Source: CAD feature listing. Evaluate the final solid. Frame: model axes, mm. A direction names the side the tool comes from. Round coordinates to 2 decimals unless told otherwise and drop trailing zeros. Write each loop counter-clockwise with the first axis right and the second up, starting at its lowest first coordinate (ties: lowest second). Pieces come first, ordered by that corner, then holes.
```python
from build123d import *

# Parameters (mm, degrees)
SKETCH1_R           = 2.15
BOSS_EXTRUDE1_DEPTH = 1.5
SKETCH3_W           = 5
SKETCH3_H           = 20
BOSS_EXTRUDE3_DEPTH = 12.5
BOSS_EXTRUDE4_REACH = 52.014


with BuildPart() as part:
    # Sketch1 → Boss-Extrude1 (new, symmetric)
    with BuildSketch(Plane(origin=(0, 0, 0), x_dir=(1, 0, 0), z_dir=(0, 1, 0))):
        with BuildLine():
            Line((-7, -6.25), (7, -6.25))
            ThreePointArc((7, -6.25), (10.535533906, -4.785533906), (12, -1.25))
            Line((12, -1.25), (12, 1.25))
            ThreePointArc((12, 1.25), (10.535533906, 4.785533906), (7, 6.25))
            Line((7, 6.25), (-7, 6.25))
            ThreePointArc((-7, 6.25), (-10.535533906, 4.785533906), (-12, 1.25))
            Line((-12, 1.25), (-12, -1.25))
            ThreePointArc((-12, -1.25), (-10.535533906, -4.785533906), (-7, -6.25))
        make_face()
        with Locations(Location((-7.25, 0, 0), (0, 0, 270))):
            Circle(SKETCH1_R, mode=Mode.SUBTRACT)
        with Locations(Location((7.25, 0, 0), (0, 0, 270))):
            Circle(SKETCH1_R, mode=Mode.SUBTRACT)
    extrude(amount=BOSS_EXTRUDE1_DEPTH, both=True)

    # Sketch3 → Boss-Extrude3 (add)
    with BuildSketch(Plane.XY.offset(6.25)):
        with Locations((0, 11.5)):
            Rectangle(SKETCH3_W, SKETCH3_H)
    extrude(amount=-BOSS_EXTRUDE3_DEPTH)

    # Sketch4 → Revolve1 (revolve)
    with BuildSketch(Plane.XY, mode=Mode.PRIVATE) as revolve1_sk:
        Polygon((-2.5, 19.5), (-22.5, 39.5), (-22.5, 60.085786438), (-21.085786438, 60.085786438), (-21.085786438, 40.085786438), (-2.5, 21.5), (0, 21.5), (0, 19.5), align=None)
    revolve(revolve1_sk.sketch.rotate(Axis((0, 0, 0), (0, 1, 0)), 56.251031305), axis=Axis((0, 0, 0), (0, 1, 0)))

    # Sketch5 → Boss-Extrude4 (add, up to next)
    with BuildSketch(Plane(origin=(0, 21.5, 0), x_dir=(1, 0, 0), z_dir=(0, 1, 0)), mode=Mode.PRIVATE) as boss_extrude4_sk1:
        with BuildLine():
            Line((2.5, -6.25), (2.5, -3.741657387))
            ThreePointArc((2.5, -3.741657387), (0, -4.5), (-2.5, -3.741657387))
            Line((-2.5, -3.741657387), (-2.5, -6.25))
            Line((-2.5, -6.25), (2.5, -6.25))
        make_face()
    boss_extrude4_tool1 = extrude(boss_extrude4_sk1.sketch, amount=BOSS_EXTRUDE4_REACH, mode=Mode.PRIVATE) - part.part
    # Sketch5 → Boss-Extrude4 (add, up to next)
    with BuildSketch(Plane(origin=(0, 21.5, 0), x_dir=(1, 0, 0), z_dir=(0, 1, 0)), mode=Mode.PRIVATE) as boss_extrude4_sk2:
        with BuildLine():
            Line((-2.5, 6.25), (-2.5, 3.741657387))
            ThreePointArc((-2.5, 3.741657387), (0, 4.5), (2.5, 3.741657387))
            Line((2.5, 3.741657387), (2.5, 6.25))
            Line((2.5, 6.25), (-2.5, 6.25))
        make_face()
    boss_extrude4_tool2 = extrude(boss_extrude4_sk2.sketch, amount=BOSS_EXTRUDE4_REACH, mode=Mode.PRIVATE) - part.part
    add(boss_extrude4_tool1.solids().sort_by_distance((0, 21.5, 5.24074))[0])
    add(boss_extrude4_tool2.solids().sort_by_distance((0, 21.5, -5.24074))[0])


solid = part.part
```
Q1. Line query: line 1 (X direction, y = 0, z = 0); line 2 (X direction, y = 53.5, z = 0). Output: solid intervals per line, ascending.
Q2. Section query D-D, the plane x = 8. Give the number of separate pieces and of enclosed holes in the cut face, and give its area (3 significant figures).
Q3. Section query B-B, the plane x = 0. Output: boundary loops of the cut face in (y, z).
Q4. Pin query (flat end, axial travel): P1, Ø2, axis at y = 24, z = 1, coming from the +X side; P2, Ø4, axis at x = -7.25, z = 0, coming from the +Y side; P3, Ø4, axis at y = 8, z = 0, coming from the +X side. Return the tip coordinate at first contact, or that it passes through.
Q5. Section query C-C, the plane y = 31.5. Output: boundary loops of the cut face in (x, z).
Q6. Section query A-A, the plane z = 0. Output: boundary loops of the cut face in (x, y).
Q7. Set-up query: faces 5 (the face through (-5, 1.5, 1)), 6 (the face through (10.57, 0.02, -4.75)), 7 (the face through (12, 0, 0)), 8 (the face through (20.48, 49.95, -5.01)). Return all of +Z, -Z, +X, -X, +Y, -Y with unobstructed straight access to the full face (end or side cutting, diameter ignored); none if empty.
Q8. Mould query, pull axis X, two halves, no side actions, for faces 1 (the face through (0, 21.5, 0)), 2 (the face through (0, 8, 6.25)), 3 (the face through (9.38, -0.02, -0.28)), 4 (the face through (-2.5, 12, 0)). Classes: pulls with the +X half, pulls with the -X half, needs draft (parallel to the pull), parting line crosses it, or undercut.
Filled in:
1. line 1: x = -12 to -9.4, -5.1 to 5.1, 9.4 to 12
1. line 2: x = -22.5 to -21.09, 21.09 to 22.5
2. separate pieces: 3
2. enclosed holes: 0
2. area: 168 mm2
3. outline: (-1.5, -6.25) - (23.25, -6.25) - (39.5, -22.5) - (60.09, -22.5) - (60.09, -21.09) - (40.09, -21.09) - (21.5, -2.5) - (21.5, 2.5) - (40.09, 21.09) - (60.09, 21.09) - (60.09, 22.5) - (39.5, 22.5) - (23.25, 6.25) - (-1.5, 6.25) - close
4. P1: stops at x = 7.94
4. P2: stops at y = 28.25
4. P3: stops at x = 2.5
5. outline: circle Ø29 at (0, 0); hole circle Ø25 at (0, 0)
6. outline: (-22.5, 39.5) - (-2.5, 19.5) - (-2.5, 1.5) - (-5.1, 1.5) - (-5.1, -1.5) - (5.1, -1.5) - (5.1, 1.5) - (2.5, 1.5) - (2.5, 19.5) - (22.5, 39.5) - (22.5, 60.09) - (21.09, 60.09) - (21.09, 40.09) - (2.5, 21.5) - (-2.5, 21.5) - (-21.09, 40.09) - (-21.09, 60.09) - (-22.5, 60.09) - close; (-12, -1.5) - (-9.4, -1.5) - (-9.4, 1.5) - (-12, 1.5) - close; (9.4, -1.5) - (12, -1.5) - (12, 1.5) - (9.4, 1.5) - close
7. face 5: +Z, -Z, -X
7. face 6: -Z, +X, -Y
7. face 7: +Z, -Z, +X, -Y
7. face 8: +Y
8. face 1: undercut
8. face 2: needs draft
8. face 3: undercut
8. face 4: pulls with the -X half
